Design review of the part built by this model. Coordinates are the model's own, in mm. A direction names the side the tool comes from. Coordinates: 2 decimals unless noted, no trailing zeros. Write each loop counter-clockwise with the first axis right and the second up, starting at its lowest first coordinate (ties: lowest second). Pieces come first, ordered by that corner, then holes.
Q1. For L1, parallel to Y at x = 12.7, z = 0.9 (3 decimals); L2, parallel to X at y = 7.5, z = 6.5 (3 decimals), list the stretches that pass through material, from the lowest coordinate up.
Q2. Take a section at A-A, the plane y = 38.1. Write out the cut boundary in (x, z) (3 decimals).
Q3. For faces 1 (the flat face through (24, 101.6, 13)), 2 (the flat face through (13, 52, 22.225)), 3 (the cylindrical face through (23.83, 40.46, 13.01)), list the 3-axis set-ups (+Z, -Z, +X, -X, +Y, -Y) from which the entire face can be reached by the end or side of a thin tool; tool diameter is ignored.
Q4. For pin 1 Ø4 at (x, y) = (12.7, 38.1) entering from +Z, flat-tipped, find the tip position at first contact; note if it passes through.
Q5. Take a section at C-C, the plane z = 1.75. Write out the cut boundary in (x, y) (3 decimals).
Q6. The part is to be moulded in two halves that separate along X. For faces 4 (the cylindrical face through (10.36, 65.646, 1.61)), 5 (the flat face through (25.4, 50, 13)), 6 (the cylindrical face through (23.83, 14.71, 11.42)), say which applies: released by +X, released by -X, zero draft, split by the parting line, or undercut.
Q7. Take a section at B-B, the plane x = 19.25. Write out the cut boundary in (y, z) (3 decimals).
Q8. Take a section at D-D, the plane y = 63.5. Write out the cut boundary in (x, z) (3 decimals), plus the area to 3 significant figures.
from build123d import *

# Parameters (mm, degrees)
SKETCH1_W           = 25.4
SKETCH1_H           = 101.6
BOSS_EXTRUDE1_DEPTH = 25.4
SHELL1_T            = -3.175
SKETCH2_R           = 3.175
CUT_EXTRUDE1_DEPTH  = 108.763073453
SKETCH3_R           = 2.38125
CUT_EXTRUDE2_DEPTH  = 7.62


with BuildPart() as part:
    # Sketch1 → Boss-Extrude1 (new body)
    with BuildSketch(Plane.XY):
        with Locations((12.7, 50.8)):
            Rectangle(SKETCH1_W, SKETCH1_H)
    extrude(amount=BOSS_EXTRUDE1_DEPTH)

    # Shell1
    shell1_openings = [part.faces().sort_by_distance(p)[0] for p in [
        (12.7, 101.6, 12.7),
        (12.7, 0, 12.7),
    ]]
    offset(amount=SHELL1_T, openings=shell1_openings, kind=Kind.INTERSECTION)

    # Sketch2 → Cut-Extrude1 (cut, through all)
    with BuildSketch(Plane.XY.offset(25.4)):
        with Locations((12.7, 12.7)):
            Circle(SKETCH2_R)
        with Locations((12.7, 38.1)):
            Circle(SKETCH2_R)
        with Locations((12.7, 88.9)):
            Circle(SKETCH2_R)
        with Locations((12.7, 63.5)):
            Circle(SKETCH2_R)
    extrude(amount=-CUT_EXTRUDE1_DEPTH, mode=Mode.SUBTRACT)

    # Sketch3 → Cut-Extrude2 (cut)
    with BuildSketch(Plane(origin=(25.4, 0, 0), x_dir=(0, 0, -1), z_dir=(1, 0, 0))):
        with Locations((-12.7, 12.7)):
            Circle(SKETCH3_R)
        with Locations((-12.7, 38.1)):
            Circle(SKETCH3_R)
    extrude(amount=-CUT_EXTRUDE2_DEPTH, mode=Mode.SUBTRACT)


solid = part.part
Responses:
1. L1: y = 0 to 9.525, 15.875 to 34.925, 41.275 to 60.325, 66.675 to 85.725, 92.075 to 101.6
1. L2: x = 0 to 3.175, 22.225 to 25.4
2. outline: (0, 0) - (9.525, 0) - (9.525, 3.175) - (3.175, 3.175) - (3.175, 22.225) - (9.525, 22.225) - (9.525, 25.4) - (0, 25.4) - close; (15.875, 0) - (25.4, 0) - (25.4, 10.319) - (22.225, 10.319) - (22.225, 3.175) - (15.875, 3.175) - close; (15.875, 22.225) - (22.225, 22.225) - (22.225, 15.081) - (25.4, 15.081) - (25.4, 25.4) - (15.875, 25.4) - close
3. face 1: +Z, -Z, +X, -X, +Y
3. face 2: +Y, -Y
3. face 3: +X
4. pin 1: passes through
5. outline: (0, 0) - (25.4, 0) - (25.4, 101.6) - (0, 101.6) - close; hole circle Ø6.35 at (12.7, 12.7); hole circle Ø6.35 at (12.7, 38.1); hole circle Ø6.35 at (12.7, 63.5); hole circle Ø6.35 at (12.7, 88.9)
6. face 4: undercut
6. face 5: released by +X
6. face 6: zero draft
7. outline: (0, 0) - (101.6, 0) - (101.6, 3.175) - (0, 3.175) - close; (0, 22.225) - (101.6, 22.225) - (101.6, 25.4) - (0, 25.4) - close
8. outline: (0, 0) - (9.525, 0) - (9.525, 3.175) - (3.175, 3.175) - (3.175, 22.225) - (9.525, 22.225) - (9.525, 25.4) - (0, 25.4) - close; (15.875, 0) - (25.4, 0) - (25.4, 25.4) - (15.875, 25.4) - (15.875, 22.225) - (22.225, 22.225) - (22.225, 3.175) - (15.875, 3.175) - close
8. area: 242 mm2
